Verification items for this drawing (mm, ordinates from the low corner). A direction names the side the tool comes from. Round coordinates to 2 decimals unless told otherwise and drop trailing zeros. Loops run counter-clockwise (first coordinate to the right, second up) from the corner with the lowest first, then second, coordinate; pieces in that order, holes last. Notation, with made-up numbers: (44, 56.5) -> (87, 56.5) arc R24 cw to (87, 77.5) -> close; hole circle Ø1 at (55, 29.25). An arc over 180 degrees is marked (long way). Use a Markdown table: item, result. Add a question column.
Q1. Material ranges on L1, parallel to Y at x = 13.75, z = 22; L2, parallel to Z at x = 5.5, y = 12.5, recorded low to high.
Q2. Sectioned sample at C-C, the plane x = 23.25. Enter the section's corners in (y, z).
Q3. Gauge pin test, flat ends, axial feed: P1, Ø2.5, axis at y = 4.5, z = 13, coming from the -X side; P2, Ø6, axis at y = 23, z = 17.5, coming from the +X side; P3, Ø4, axis at x = 4, z = 19, coming from the -Y side. Record the tip position at first contact, or that the pin passes through.
Q4. Sectioned sample at D-D, the plane z = 15.5. Enter the section's corners in (x, y).
Q5. Sectioned sample at B-B, the plane z = 19. Enter the section's corners in (x, y).
Q6. Set-up check for the marked faces 1, 2 and 3: record each of +Z, -Z, +X, -X, +Y, -Y from which the full face is reachable in a straight line by a thin tool's end or side.
Q7. Sectioned sample at A-A, the plane y = 14.75. Enter the section's corners in (x, z).
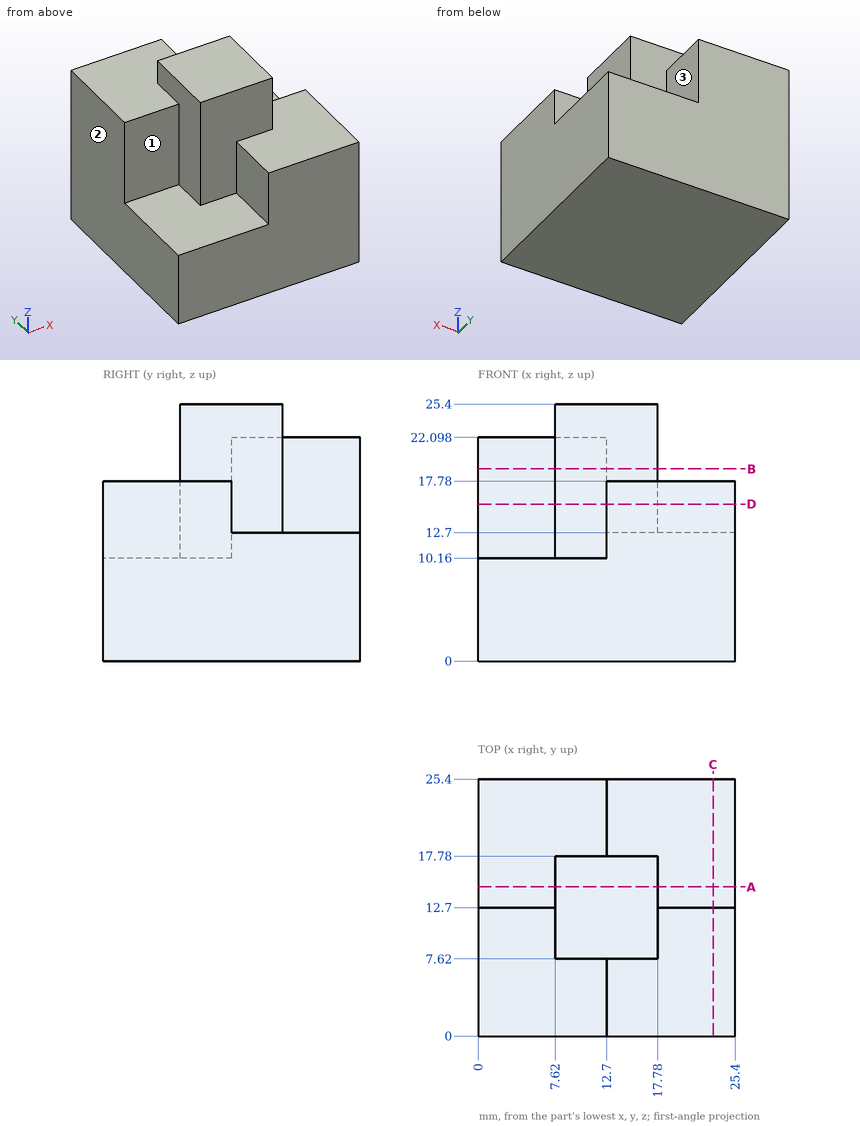
Values:
| question | item | result |
|---|---|---|
| 1 | L1 | 7.62 to 17.78 |
| 1 | L2 | 0 to 10.16 |
| 2 | outline | (0, 0) -> (25.4, 0) -> (25.4, 12.7) -> (12.7, 12.7) -> (12.7, 17.78) -> (0, 17.78) -> close |
| 3 | P1 | x = 12.7 |
| 3 | P2 | x = 12.7 |
| 3 | P3 | y = 12.7 |
| 4 | outline | (0, 12.7) -> (7.62, 12.7) -> (7.62, 7.62) -> (12.7, 7.62) -> (12.7, 0) -> (25.4, 0) -> (25.4, 12.7) -> (17.78, 12.7) -> (17.78, 17.78) -> (12.7, 17.78) -> (12.7, 25.4) -> (0, 25.4) -> close |
| 5 | outline | (0, 12.7) -> (7.62, 12.7) -> (7.62, 7.62) -> (17.78, 7.62) -> (17.78, 17.78) -> (12.7, 17.78) -> (12.7, 25.4) -> (0, 25.4) -> close |
| 6 | face 1 | +Z, -X, -Y |
| 6 | face 2 | +Z, -Z, -X, +Y, -Y |
| 6 | face 3 | +Z, +X, +Y |
| 7 | outline | (0, 0) -> (25.4, 0) -> (25.4, 12.7) -> (17.78, 12.7) -> (17.78, 25.4) -> (7.62, 25.4) -> (7.62, 22.1) -> (0, 22.1) -> close |
